Autodesk Inventor part; units mm, degrees
ref_plane "YZ Plane" through (0, 0, 0) normal (1, 0, 0) x (0, 1, 0)
ref_plane "XZ Plane" through (0, 0, 0) normal (0, 1, 0) x (-1, 0, 0)
ref_plane "XY Plane" through (0, 0, 0) normal (0, 0, 1) x (1, 0, 0)
sketch "Skizze1" plane through (0, 0, 0) normal (0, 0, 1) x (1, 0, 0)
  circle A0 centre (0, 0) radius 17.5
  dimension "d0" = 35
extrude "Extrusion1" add sketch "Skizze1" against normal blind 22
sketch "Skizze2" plane through (0, 0, -22) normal (0, 0, -1) x (-1, 0, 0)
  circle A0 centre (0, 0) radius 17.5
  circle A1 centre (0, 0) radius 18
  dimension "d3" = 36
extrude "Extrusion2" add sketch "Skizze2" along normal blind 57.1 contours A0 | A1
sketch "Skizze3" plane through (0, 0, 0) normal (0, 0, 1) x (1, 0, 0)
  circle A0 centre (0, 0) radius 17.5
  circle A1 centre (0, 7) radius 6
  line L0 (0, 0) -> (0, 7) construction
  dimension "d6" = 12
  dimension "d7" = 7
extrude "Extrusion3" add sketch "Skizze3" along normal blind 10 contours A1
sketch "Skizze4" plane through (0, 7, 10) normal (0, 0, 1) x (1, 0, 0)
  circle A0 centre (0, 0) radius 6
  circle A1 centre (0, 0) radius 3
  point P0 (0, -7)
  dimension "d10" = 6
extrude "Extrusion4" add sketch "Skizze4" along normal blind 17 contours A1
ref_plane "Arbeitsebene1" through (0, 7, 10) normal (1, 0, 0) x (0, 0, 1)
sketch "Skizze5" plane through (0, 0, 0) normal (0, 0, 1) x (1, 0, 0)
  circle A0 centre (0, 0) radius 17.5
  circle A1 centre (0, 0) radius 15.5 construction
  line L0 (0, 0) -> (0, -17.5) construction
  line L1 (0, 0) -> (-15.1554, 8.75) construction
  line L2 (0, 0) -> (15.1554, 8.75) construction
  point P0 (-13.4234, 7.75)
  point P1 (13.4234, 7.75)
  point P2 (0, -15.5)
  dimension "d13" = 120
  dimension "d14" = 120
  dimension "d15" = 31
hole "Bohrung1" at (-13.4234, 7.75, 0) at (13.4234, 7.75, 0) at (0, -15.5, 0) direction (0, 0, -1) diameter 2 depth 8
equation "\"d14\" = d13"
properties part number "Conrad Motor" material "Eisen, grau"
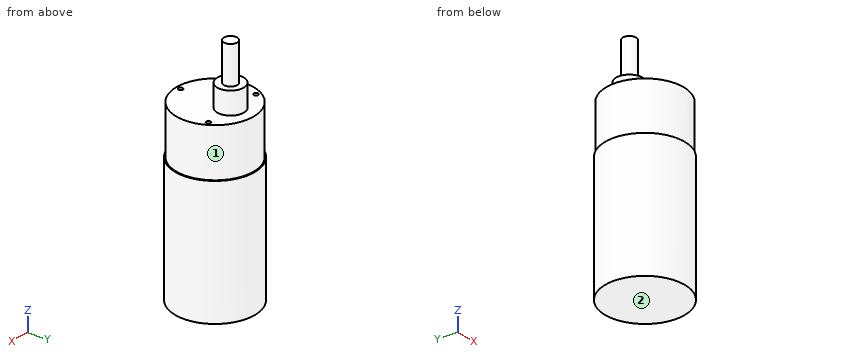
CAD build for the part. Positions are in the model's coordinates, mm. Face numbers are marked on the shaded views. A direction names the side the tool comes from. Give positions to 0.01 mm unless a question says otherwise; leave off trailing zeros. Write each loop counter-clockwise with the first axis right and the second up, starting at its lowest first coordinate (ties: lowest second). Pieces come first, ordered by that corner, then holes. Notation, with made-up numbers: M -18.5,-10.5 L 18.5,-10.5 A32 cw 18.5,17.5 Z; hole C 88.5,38.5 d3. An arc over 180 degrees is marked long. Put each result on its own line as item: value. Start each with the question number.
(1) Band-saw the part on B-B, the plane y = 0. Write the cut outline in (x, z), and give its area (3 significant figures).
(2) Band-saw the part on A-A, the plane x = 0. Write the cut outline in (y, z).
(3) Flat gauge pins, fed straight in: pin 1 Ø6 at (y, z) = (6.5, -57.5) entering from -X; pin 2 Ø6 at (x, y) = (3.5, -12.5) entering from +Z; pin 3 Ø3 at (x, z) = (-0.5, -13) entering from -Y. Where does each tip first touch, or does it go through?
(4) Band-saw the part on D-D, the plane x = 7. Write the cut outline in (y, z), and give its area (3 significant figures).
(5) Which spindle directions (+Z, -Z, +X, -X, +Y, -Y) get a long thin tool onto all of the face, cutting with end or side? Do the marked faces 1 and 2. Say none if no direction does.
(6) Probe L1, parallel to Y at x = 0, z = -2; L2, parallel to X at y = 7, z = -3; L3, parallel to Z at x = -14.5, y = 0.5. List the from-to ranges inside material, lowest first.
(7) Band-saw the part on C-C, the plane z = 7.5. Write the cut outline in (x, y).
Response values:
1. outline: M -18,-79.1 L 18,-79.1 L 18,-22 L 17.5,-22 L 17.5,0 L -17.5,0 L -17.5,-22 L -18,-22 Z
1. area: 2,830 mm2
2. outline: M -18,-79.1 L 18,-79.1 L 18,-22 L 17.5,-22 L 17.5,0 L 13,0 L 13,10 L 10,10 L 10,27 L 4,27 L 4,10 L 1,10 L 1,0 L -14.5,0 L -14.5,-8 L -16.5,-8 L -16.5,0 L -17.5,0 L -17.5,-22 L -18,-22 Z
3. pin 1: stops at x = -17.66
3. pin 2: stops at z = 0
3. pin 3: stops at y = -17.5
4. outline: M -16.58,-79.1 L 16.58,-79.1 L 16.58,-22 L 16.04,-22 L 16.04,0 L -16.04,0 L -16.04,-22 L -16.58,-22 Z
4. area: 2,600 mm2
5. face 1: +Z
5. face 2: -Z, +X, -X, +Y, -Y
6. L1: y = -17.5 to -16.5, -14.5 to 17.5
6. L2: x = -16.04 to -14.08, -12.76 to 12.76, 14.08 to 16.04
6. L3: z = -79.1 to 0
7. outline: C 0,7 d12
